Geometry check sheet. Reference: the model listing, model coordinates, mm. A direction names the side the tool comes from. Give positions to 0.01 mm unless a question says otherwise; leave off trailing zeros. Write each loop counter-clockwise with the first axis right and the second up, starting at its lowest first coordinate (ties: lowest second). Pieces come first, ordered by that corner, then holes. Notation, with made-up numbers: (77, -35) -> (81, -35) arc R25 ccw to (81, -7) -> close; hole circle Ø9 at (15, 67). An arc over 180 degrees is marked (long way). Write item = value, one per line. Start each with the question number.
1. Cross-section at B-B, the plane z = 23.5. Record the cut outline in (x, y).
2. Cross-section at D-D, the plane y = -24. Record the cut outline in (x, z).
3. Cross-section at A-A, the plane z = 8. Record the cut outline in (x, y), plus the area to 3 significant figures.
4. Mould release check, pull along X, two halves, no side actions. Record for faces 1 (the cylindrical face through (36.47, -39.14, 0.9)), 2 (the cylindrical face through (33.14, 0.9, 2.46)), 3 (the cylindrical face through (26.54, -12, 2.46)), 4 (the cylindrical face through (3.294, -6.308, 2.465)): pulls with the +X half, pulls with the -X half, needs draft (parallel to the pull), parting line crosses it, or undercut.
5. Thickness scan on line 1 along Y through (x, z) = (5, 1); line 2 along Y through (x, z) = (36.65, 39); line 3 along Z through (x, y) = (36, -30). Record the ranges inside material, lowest first.
6. Set-up check for faces 5 (the flat face through (17, -30, 3)), 6 (the flat face through (39, -15, 13)), 7 (the flat face through (9, -7, 5)): record each of +Z, -Z, +X, -X, +Y, -Y from which the full face is reachable in a straight line by a thin tool's end or side.
7. Depth check by flat-ended pin: P1, Ø23, axis at x = 17, y = -15, coming from the +Z side; P2, Ø3.5, axis at x = 5, y = -25, coming from the +Z side; P3, Ø1, axis at y = -4.5, z = 23, coming from the -X side; P4, Ø2.5, axis at x = 11, z = 2, coming from the +Y side. Enter the tip coordinate at first touch or a pass-through.
8. Cross-section at C-C, the plane x = 29. Record the cut outline in (y, z), plus the area to 3 significant figures.
```python
from build123d import *

# Parameters (mm, degrees)
SKETCH2_W           = 34
SKETCH2_H           = 30
SKETCH2_R           = 10
SKETCH2_R_2         = 2.15
BOSS_EXTRUDE1_DEPTH = 5
SKETCH6_W           = 5
SKETCH6_H           = 50
BOSS_EXTRUDE3_DEPTH = 40
SKETCH10_W          = 5
SKETCH10_H          = 30
BOSS_EXTRUDE4_DEPTH = 5
SKETCH11_W          = 5
SKETCH11_H          = 10
BOSS_EXTRUDE5_DEPTH = 5
FILLET3_R           = 3
FILLET4_R           = 3
FILLET5_R           = 3
SKETCH12_R          = 2.15
SKETCH12_R_2        = 10
CUT_EXTRUDE3_DEPTH  = 5


with BuildPart() as part:
    # Sketch2 → Boss-Extrude1 (new body)
    with BuildSketch(Plane.XY):
        with Locations((17, -15)):
            Rectangle(SKETCH2_W, SKETCH2_H)
        with Locations((17, -15)):
            Circle(SKETCH2_R, mode=Mode.SUBTRACT)
        with Locations((29, -5)):
            Circle(SKETCH2_R_2, mode=Mode.SUBTRACT)
        with Locations((5, -5)):
            Circle(SKETCH2_R_2, mode=Mode.SUBTRACT)
        with Locations((5, -25)):
            Circle(SKETCH2_R_2, mode=Mode.SUBTRACT)
        with Locations((29, -25)):
            Circle(SKETCH2_R_2, mode=Mode.SUBTRACT)
    extrude(amount=BOSS_EXTRUDE1_DEPTH)



with BuildPart() as body_2:
    # Sketch6 → Boss-Extrude3 (new body)
    with BuildSketch(Plane.XY.offset(5)):
        with Locations((36.5, -15)):
            Rectangle(SKETCH6_W, SKETCH6_H)
    extrude(amount=BOSS_EXTRUDE3_DEPTH)


with BuildPart() as part_1:
    add(part.part)

    add(body_2.part)  # Boss-Extrude4 merges body 2
    # Sketch10 → Boss-Extrude4 (add)
    with BuildSketch(Plane(origin=(34, 0, 0), x_dir=(0, 0, -1), z_dir=(1, 0, 0))):
        with Locations((-2.5, -15)):
            Rectangle(SKETCH10_W, SKETCH10_H)
    extrude(amount=BOSS_EXTRUDE4_DEPTH)

    # Sketch11 → Boss-Extrude5 (add)
    with BuildSketch(Plane(origin=(0, 0, 5), x_dir=(-1, 0, 0), z_dir=(0, 0, -1))):
        with Locations((-36.5, -35)):
            Rectangle(SKETCH11_W, SKETCH11_H)
        with Locations((-36.5, 5)):
            Rectangle(SKETCH11_W, SKETCH11_H)
    extrude(amount=BOSS_EXTRUDE5_DEPTH)

    # Fillet3
    fillet3_edges = [part_1.edges().sort_by_distance(p)[0] for p in [
        (34, -30, 2.5),
        (34, 0, 2.5),
        (0, -30, 2.5),
        (0, 0, 2.5),
    ]]
    fillet(fillet3_edges, radius=FILLET3_R)

    # Fillet4
    fillet4_edges = [part_1.edges().sort_by_distance(p)[0] for p in [
        (36.5, -40, 0),
    ]]
    fillet(fillet4_edges, radius=FILLET4_R)

    # Fillet5
    fillet5_edges = [part_1.edges().sort_by_distance(p)[0] for p in [
        (36.5, -40, 45),
        (36.5, 10, 45),
        (36.5, 10, 0),
    ]]
    fillet(fillet5_edges, radius=FILLET5_R)

    # Sketch12 → Cut-Extrude3 (cut)
    with BuildSketch(Plane(origin=(39, 0, 0), x_dir=(0, 0, -1), z_dir=(1, 0, 0))):
        with Locations((-39, 0.5)):
            Circle(SKETCH12_R)
        with Locations((-23.5, -15)):
            Circle(SKETCH12_R_2)
        with Locations((-8, 0.5)):
            Circle(SKETCH12_R)
        with Locations((-8, -30.5)):
            Circle(SKETCH12_R)
        with Locations((-39, -30.5)):
            Circle(SKETCH12_R)
    extrude(amount=-CUT_EXTRUDE3_DEPTH, mode=Mode.SUBTRACT)


solid = part_1.part
```
Answers:
q1.outline = (34, -40) -> (39, -40) -> (39, -25) -> (34, -25) -> close; (34, -5) -> (39, -5) -> (39, 10) -> (34, 10) -> close
q2.outline = (0, 0) -> (3.1, 0) -> (3.1, 5) -> (0, 5) -> close; (6.9, 0) -> (12.64, 0) -> (12.64, 5) -> (6.9, 5) -> close; (21.36, 0) -> (27.1, 0) -> (27.1, 5) -> (21.36, 5) -> close; (30.9, 0) -> (39, 0) -> (39, 19.14) -> (34, 19.14) -> (34, 5) -> (30.9, 5) -> close; (34, 27.86) -> (39, 27.86) -> (39, 45) -> (34, 45) -> close
q3.outline = (34, -40) -> (39, -40) -> (39, -32.65) -> (34, -32.65) -> close; (34, -28.35) -> (39, -28.35) -> (39, -1.65) -> (34, -1.65) -> close; (34, 2.65) -> (39, 2.65) -> (39, 10) -> (34, 10) -> close
q3.area = 207 mm^2
q4.face_1 = needs draft
q4.face_2 = pulls with the -X half
q4.face_3 = undercut
q4.face_4 = undercut
q5.line_1 = -30 to -27.15, -22.85 to -7.15, -2.85 to 0
q5.line_2 = -40 to -32.65, -28.35 to -1.65, 2.65 to 10
q5.line_3 = 0 to 5.91, 10.09 to 36.91, 41.09 to 45
q6.face_5 = +Z, -Z, -X, -Y
q6.face_6 = +Z, -Z, +X, +Y, -Y
q6.face_7 = +Z, -X, +Y, -Y
q7.P1 = 5
q7.P2 = through
q7.P3 = 34
q7.P4 = 0
q8.outline = (-30, 0) -> (-27.15, 0) -> (-27.15, 5) -> (-30, 5) -> close; (-22.85, 0) -> (-7.15, 0) -> (-7.15, 5) -> (-22.85, 5) -> close; (-2.85, 0) -> (0, 0) -> (0, 5) -> (-2.85, 5) -> close
q8.area = 107 mm^2
